The model under review builds one solid part; all positions refer to its coordinate system, in mm. Face numbers are marked on the shaded views. Round coordinates to 2 decimals unless told otherwise and drop trailing zeros. Order: outer loops, then holes, each group sorted by start corner. A loop starts at its lowest first (then second) coordinate and runs counter-clockwise, first axis right, second up. Notation, with made-up numbers: (58, 38) -> (84, 38) arc R31 cw to (84, 63) -> close; hole circle Ø5 at (9, -1). An arc over 180 degrees is marked (long way). Return JSON: item names as keys, results as strings. Group by question number.
from build123d import *

# Parameters (mm, degrees)
SALIENTE_EXTRUIR1_DEPTH = 4
CROQUIS1_3_R            = 4
SALIENTE_EXTRUIR2_DEPTH = 6
SALIENTE_EXTRUIR3_DEPTH = 4
MATRIZC1_COUNT          = 36
FILLET1_R               = 3.175


with BuildPart() as part:
    # Croquis1 → Saliente-Extruir1 (new body)
    with BuildSketch(Plane(origin=(0, 0, 0), x_dir=(1, 0, 0), z_dir=(0, 1, 0))):
        with BuildLine():
            Line((-7.5, 76.2), (-7.5, 0))
            ThreePointArc((-7.5, 0), (0, -7.5), (7.5, 0))
            Line((7.5, 0), (7.5, 76.2))
            Line((7.5, 76.2), (-7.5, 76.2))
        make_face()
        with BuildLine():
            ThreePointArc((-3.175, 68.58), (0, 71.755), (3.175, 68.58))
            Line((3.175, 68.58), (3.175, 17.78))
            ThreePointArc((3.175, 17.78), (0, 14.605), (-3.175, 17.78))
            Line((-3.175, 17.78), (-3.175, 68.58))
        make_face(mode=Mode.SUBTRACT)
        with BuildLine():
            ThreePointArc((-2.954423259, 0.520944533), (2.974334584, -0.391578577), (-2.988584094, 0.261467228))
            ThreePointArc((-2.988584094, 0.261467228), (-2.974334584, 0.391578577), (-2.954423259, 0.520944533))
        make_face(mode=Mode.SUBTRACT)
    extrude(amount=SALIENTE_EXTRUIR1_DEPTH)

    # Croquis1_3 → Saliente-Extruir2 (add)
    with BuildSketch(Plane(origin=(0, 0, 0), x_dir=(1, 0, 0), z_dir=(0, 1, 0))):
        with BuildLine():
            Line((-7.5, 76.2), (-7.5, 0))
            ThreePointArc((-7.5, 0), (0, -7.5), (7.5, 0))
            Line((7.5, 0), (7.5, 76.2))
            Line((7.5, 76.2), (-7.5, 76.2))
        make_face()
        with BuildLine():
            ThreePointArc((-3.175, 68.58), (0, 71.755), (3.175, 68.58))
            Line((3.175, 68.58), (3.175, 17.78))
            ThreePointArc((3.175, 17.78), (0, 14.605), (-3.175, 17.78))
            Line((-3.175, 17.78), (-3.175, 68.58))
        make_face(mode=Mode.SUBTRACT)
        with Locations(Location((0, 0, 0), (0, 0, 270))):
            Circle(CROQUIS1_3_R, mode=Mode.SUBTRACT)
    extrude(amount=SALIENTE_EXTRUIR2_DEPTH)

    # Croquis1_4 → Saliente-Extruir3 (add)
    with BuildSketch(Plane(origin=(0, 0, 0), x_dir=(1, 0, 0), z_dir=(0, 1, 0))):
        with BuildLine():
            Line((-3, 0), (-2.73953542, 0.239678293))
            Line((-2.73953542, 0.239678293), (-2.988584094, 0.261467228))
            ThreePointArc((-2.988584094, 0.261467228), (-2.997144665, 0.130858162), (-3, 0))
        make_face()
        with BuildLine():
            Line((-2.988584094, 0.261467228), (-2.73953542, 0.239678293))
            Line((-2.73953542, 0.239678293), (-2.954423259, 0.520944533))
            ThreePointArc((-2.954423259, 0.520944533), (-2.974334584, 0.391578577), (-2.988584094, 0.261467228))
        make_face()
    saliente_extruir3 = extrude(amount=SALIENTE_EXTRUIR3_DEPTH)

    # MatrizC1: Saliente-Extruir3 ×36 about axis
    matrizc1_axis = Axis((0, 0, 0), (0, 1, 0))
    for i in range(1, MATRIZC1_COUNT):
        add(saliente_extruir3.rotate(matrizc1_axis, i * 360 / MATRIZC1_COUNT))

    # Fillet1
    fillet1_edges = [part.edges().sort_by_distance(p)[0] for p in [
        (-7.5, 3, -76.2),
        (7.5, 3, -76.2),
    ]]
    fillet(fillet1_edges, radius=FILLET1_R)


solid = part.part
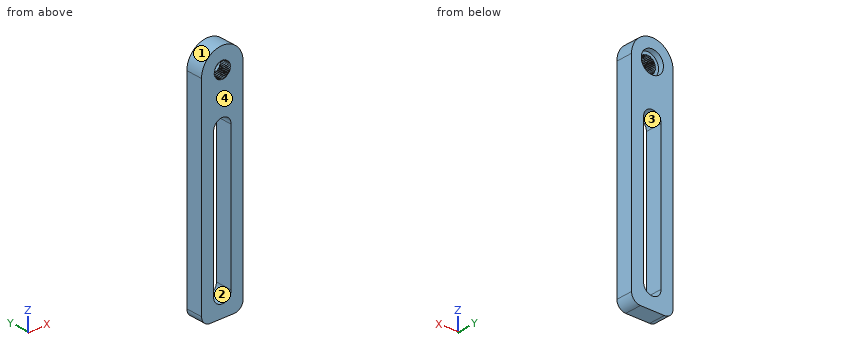
Item 1: Consider section A-A on z = -47.5. State the section outline as (x, y) points (3 decimals), plus the area to 3 significant figures.
Item 2: Insertion check: pin 1 Ø1.5 at (x, y) = (-1.5, 4) entering from +Z; pin 2 Ø1 at (x, y) = (-2, 3) entering from +Z; pin 3 Ø1.5 at (x, y) = (3.5, 2) entering from +Z. Each pin has a flat end and moves straight along its axis. Give the tip position at first contact, or say it passes through.
Item 3: Consider section B-B on y = 1.35. Give the number of separate pieces and of enclosed holes in the cut face, plus the area to 3 significant figures.
Item 4: Wall thickness on line 1 along Z through (x, y) = (0, 4.95) (3 decimals); line 2 along X through (y, z) = (2.8, -39) (3 decimals); line 3 along Z through (x, y) = (2.25, 4.85): over which ranges is each line inside the solid? List them lowest first.
Item 5: The part is to be moulded in two halves that separate along X. For the marked faces 1, 2, 3 and 4, say which applies: +X half, -X half, draft (parallel to the pull), parting line (faces both ways), or undercut.
Values:
{
 "1": {"outline": "(-7.5, 0) -> (-3.175, 0) -> (-3.175, 6) -> (-7.5, 6) -> close; (3.175, 0) -> (7.5, 0) -> (7.5, 6) -> (3.175, 6) -> close", "area": "51.9 mm^2"},
 "2": {"pin 1": "z = 7.46", "pin 2": "z = 7.35", "pin 3": "z = 6.98"},
 "3": {"separate pieces": "1", "enclosed holes": "2", "area": "847 mm^2"},
 "4": {"line 1": "-76.2 to -71.755, -14.605 to -4, 4 to 7.5", "line 2": "-7.5 to -3.175, 3.175 to 7.5", "line 3": "-76.2 to -70.82, -15.54 to -3.31, 3.31 to 7.15"},
 "5": {"face 1": "parting line", "face 2": "undercut", "face 3": "undercut", "face 4": "draft"}
}
